Design review of the part built by this model. Coordinates are the model's own, in mm. A direction names the side the tool comes from. Round coordinates to 2 decimals unless told otherwise and drop trailing zeros. Order: outer loops, then holes, each group sorted by start corner. A loop starts at its lowest first (then second) coordinate and runs counter-clockwise, first axis right, second up.
from build123d import *

# Parameters (mm, degrees)
SKETCH_2_R      = 2.66
SKETCH_2_R_2    = 1.5
EXTRUDE_1_DEPTH = 1.5
SKETCH_3_R      = 6
SKETCH_3_R_2    = 4.25
EXTRUDE_2_DEPTH = 5


with BuildPart() as part:
    # 草图2 → 凸台-拉伸1 (new body)
    with BuildSketch(Plane.XY):
        with BuildLine():
            Line((-5.188427748, -15.986660076), (-20.8, -15.986660076))
            ThreePointArc((-20.8, -15.986660076), (-21.507106781, -16.279553295), (-21.8, -16.986660076))
            Line((-21.8, -16.986660076), (-21.8, -21))
            ThreePointArc((-21.8, -21), (-21.507106781, -21.707106781), (-20.8, -22))
            Line((-20.8, -22), (-5.196152423, -22))
            ThreePointArc((-5.196152423, -22), (0, -25), (5.196152423, -22))
            Line((5.196152423, -22), (20.8, -22))
            ThreePointArc((20.8, -22), (21.507106781, -21.707106781), (21.8, -21))
            Line((21.8, -21), (21.8, -16.986660076))
            ThreePointArc((21.8, -16.986660076), (21.507106781, -16.279553295), (20.8, -15.986660076))
            Line((20.8, -15.986660076), (5.188427748, -15.986660076))
            ThreePointArc((5.188427748, -15.986660076), (4.237187139, -14.751912766), (3, -13.803847577))
            Line((3, -13.803847577), (3, 1.8))
            ThreePointArc((3, 1.8), (2.707106781, 2.507106781), (2, 2.8))
            Line((2, 2.8), (-2, 2.8))
            ThreePointArc((-2, 2.8), (-2.707106781, 2.507106781), (-3, 1.8))
            Line((-3, 1.8), (-3, -13.803847577))
            ThreePointArc((-3, -13.803847577), (-4.237187139, -14.751912766), (-5.188427748, -15.986660076))
        make_face()
        with Locations((0, -19)):
            Circle(SKETCH_2_R, mode=Mode.SUBTRACT)
        with Locations((-18.8, -19)):
            Circle(SKETCH_2_R_2, mode=Mode.SUBTRACT)
        with Locations((18.8, -19)):
            Circle(SKETCH_2_R_2, mode=Mode.SUBTRACT)
        with Locations((0, -0.2)):
            Circle(SKETCH_2_R_2, mode=Mode.SUBTRACT)
    extrude(amount=EXTRUDE_1_DEPTH)

    # 草图3 → 凸台-拉伸2 (add)
    with BuildSketch(Plane.XY.offset(1.5)):
        with Locations(Location((0, -19, 0), (0, 0, 210))):
            Circle(SKETCH_3_R)
        with Locations((0, -19)):
            Circle(SKETCH_3_R_2, mode=Mode.SUBTRACT)
    extrude(amount=EXTRUDE_2_DEPTH)


solid = part.part
1) Take a section at D-D on z = 4.5. Give the boundary of the cut face in (x, y).
Results:
outline: circle Ø12 at (0, -19); hole circle Ø8.5 at (0, -19)
2) To check wall thickness, follow line 1 along Y through (x, z) = (-18.8, 1.1); line 2 along Y through (x, z) = (0, 0.7); line 3 along Y through (x, z) = (0, 4.2). State the ranges of each line that lie inside material, in increasing order.
Results:
line 1: y = -22 to -20.5, -17.5 to -15.99
line 2: y = -25 to -21.66, -16.34 to -1.7, 1.3 to 2.8
line 3: y = -25 to -23.25, -14.75 to -13
3) Take a section at B-B on x = 18.8. Give the boundary of the cut face in (y, z).
Results:
outline: (-22, 0) - (-20.5, 0) - (-20.5, 1.5) - (-22, 1.5) - close; (-17.5, 0) - (-15.99, 0) - (-15.99, 1.5) - (-17.5, 1.5) - close
4) Take a section at C-C on y = -19. Give the boundary of the cut face in (x, z), plus the area to 3 significant figures.
Results:
outline: (-21.8, 0) - (-20.3, 0) - (-20.3, 1.5) - (-21.8, 1.5) - close; (-17.3, 0) - (-2.66, 0) - (-2.66, 1.5) - (-4.25, 1.5) - (-4.25, 6.5) - (-6, 6.5) - (-6, 1.5) - (-17.3, 1.5) - close; (2.66, 0) - (17.3, 0) - (17.3, 1.5) - (6, 1.5) - (6, 6.5) - (4.25, 6.5) - (4.25, 1.5) - (2.66, 1.5) - close; (20.3, 0) - (21.8, 0) - (21.8, 1.5) - (20.3, 1.5) - close
area: 65.9 mm2
5) The part is to be moulded in two halves that separate along X. For faces 1 (the face through (-0.325, -1.664, 0.74)), 2 (the face through (-21.5, -16.27, 0.74)), 3 (the face through (13, -22, 1)), 4 (the face through (21.8, -19, 1)), say which applies: released by +X, released by -X, zero draft, split by the parting line, or undercut.
Results:
face 1: undercut
face 2: released by -X
face 3: zero draft
face 4: released by +X
6) For faces 5 (the face through (3, -6, 1)), 6 (the face through (-13, -22, 1)), 7 (the face through (-4, -17, 6.5)), 8 (the face through (-2, -21, 1.5)), list the 3-axis set-ups (+Z, -Z, +X, -X, +Y, -Y) from which the entire face can be reached by the end or side of a thin tool; tool diameter is ignored.
Results:
face 5: +Z, -Z, +X, +Y
face 6: +Z, -Z, -X, -Y
face 7: +Z, +X, -X, +Y, -Y
face 8: +Z
7) Clearance check with flat-ended pins moving along their axes: P1, Ø3, axis at x = 5.5, z = 4.5, coming from the -Y side; P2, Ø1.5, axis at x = -11.5, y = -20, coming from the +Z side; P3, Ø2.5, axis at x = 0, y = -0.2, coming from the -Z side; P4, Ø1.2, axis at x = 10, z = 1, coming from the +Y side. State where each tip first meets the part, or that it passes through.
Results:
P1: stops at y = -23.47
P2: stops at z = 1.5
P3: passes through
P4: stops at y = -15.99
8) Take a section at A-A on y = -0.2. Give the boundary of the cut face in (x, z), plus the area to 3 significant figures.
Results:
outline: (-3, 0) - (-1.5, 0) - (-1.5, 1.5) - (-3, 1.5) - close; (1.5, 0) - (3, 0) - (3, 1.5) - (1.5, 1.5) - close
area: 4.50 mm2
